Can you work these out from the model? Positions are in its coordinate system, mm. Face numbers are marked on the shaded views. Round coordinates to 2 decimals unless told otherwise and drop trailing zeros. Order: outer loops, then holes, each group sorted by start corner. A loop starts at its lowest first (then second) coordinate and runs counter-clockwise, first axis right, second up.
Q1. Will these pins go through, and if not, where does the flat tip stop? P1, Ø2, axis at x = -25, y = 5.5, coming from the +Z side (3 decimals); P2, Ø2, axis at x = 39, z = -13, coming from the -Y side; P3, Ø1, axis at x = 45, y = 1.5, coming from the -Z side (3 decimals); P4, Ø1, axis at x = -48, y = 2, coming from the +Z side (3 decimals).
Q2. If we section it at A-A (x = 22): Please give me the cut outline in (y, z) (3 decimals), plus the area to 3 significant figures.
Q3. If I drill on line 1 (X direction, y = 1.75, z = 24.5) (3 decimals); line 2 (Z direction, x = 4, y = 5.75) (3 decimals); line 3 (Z direction, x = -42.5, y = 4) (3 decimals), over which ranges is the centre line in solid material (lowest first)?
Q4. If we section it at B-B (y = 5.5): Please give me the cut outline in (x, z) (3 decimals), plus the area to 3 significant figures.
Q5. If we section it at D-D (x = 6): Please give me the cut outline in (y, z) (3 decimals), plus the area to 3 significant figures.
Q6. If we section it at C-C (z = -14): Please give me the cut outline in (x, y) (3 decimals), plus the area to 3 significant figures.
Q7. We'd pull the mould along Z, two halves only. Please class the marked faces 1 and 2: pulls with the +Z half, pulls with the -Z half, needs draft (parallel to the pull), parting line crosses it, or undercut.
from build123d import *

# Parameters (mm, degrees)
SKETCH1_W           = 7.75
SKETCH1_H           = 32.45
SKETCH1_H_2         = 7.9
SKETCH1_H_3         = 7.75
SKETCH1_W_2         = 16.15
SKETCH1_W_3         = 15.85
BOSS_EXTRUDE1_DEPTH = 3.2
SKETCH2_W           = 127.65
SKETCH2_H           = 6
BOSS_EXTRUDE2_DEPTH = 1
SKETCH3_W           = 127.65
SKETCH3_H           = 2.4
BOSS_EXTRUDE3_DEPTH = 5.4


with BuildPart() as part:
    # Sketch1 → Boss-Extrude1 (new body)
    with BuildSketch(Plane(origin=(0, 0, 0), x_dir=(1, 0, 0), z_dir=(0, 1, 0))):
        with Locations((-59.95, 0)):
            Rectangle(SKETCH1_W, SKETCH1_H)
        with Locations((-59.95, 20.175)):
            Rectangle(SKETCH1_W, SKETCH1_H_2)
        with Locations((-59.95, 28)):
            Rectangle(SKETCH1_W, SKETCH1_H_3)
        with Locations((-59.95, -20.175)):
            Rectangle(SKETCH1_W, SKETCH1_H_2)
        with Locations((-59.95, -28)):
            Rectangle(SKETCH1_W, SKETCH1_H_3)
        with Locations((-48, 20.175)):
            Rectangle(SKETCH1_W_2, SKETCH1_H_2)
        with Locations((-48, -20.175)):
            Rectangle(SKETCH1_W_2, SKETCH1_H_2)
        with Locations((-32, -28)):
            Rectangle(SKETCH1_W_3, SKETCH1_H_3)
        with Locations((-32, -20.175)):
            Rectangle(SKETCH1_W_3, SKETCH1_H_2)
        with Locations((-32, 0)):
            Rectangle(SKETCH1_W_3, SKETCH1_H)
        with Locations((-32, 20.175)):
            Rectangle(SKETCH1_W_3, SKETCH1_H_2)
        with Locations((-32, 28)):
            Rectangle(SKETCH1_W_3, SKETCH1_H_3)
        with Locations((-16, 20.175)):
            Rectangle(SKETCH1_W_2, SKETCH1_H_2)
        with Locations((-16, -20.175)):
            Rectangle(SKETCH1_W_2, SKETCH1_H_2)
        with Locations((0, -20.175)):
            Rectangle(SKETCH1_W_3, SKETCH1_H_2)
        with Locations((0, -28)):
            Rectangle(SKETCH1_W_3, SKETCH1_H_3)
        with Locations((0, 20.175)):
            Rectangle(SKETCH1_W_3, SKETCH1_H_2)
        Rectangle(SKETCH1_W_3, SKETCH1_H)
        with Locations((0, 28)):
            Rectangle(SKETCH1_W_3, SKETCH1_H_3)
        with Locations((32, 28)):
            Rectangle(SKETCH1_W_3, SKETCH1_H_3)
        with Locations((32, 20.175)):
            Rectangle(SKETCH1_W_3, SKETCH1_H_2)
        with Locations((32, 0)):
            Rectangle(SKETCH1_W_3, SKETCH1_H)
        with Locations((32, -20.175)):
            Rectangle(SKETCH1_W_3, SKETCH1_H_2)
        with Locations((32, -28)):
            Rectangle(SKETCH1_W_3, SKETCH1_H_3)
        with Locations((16, 20.175)):
            Rectangle(SKETCH1_W_2, SKETCH1_H_2)
        with Locations((16, -20.175)):
            Rectangle(SKETCH1_W_2, SKETCH1_H_2)
        with Locations((48, -20.175)):
            Rectangle(SKETCH1_W_2, SKETCH1_H_2)
        with Locations((48, 20.175)):
            Rectangle(SKETCH1_W_2, SKETCH1_H_2)
        with Locations((59.95, 28)):
            Rectangle(SKETCH1_W, SKETCH1_H_3)
        with Locations((59.95, 20.175)):
            Rectangle(SKETCH1_W, SKETCH1_H_2)
        with Locations((59.95, 0)):
            Rectangle(SKETCH1_W, SKETCH1_H)
        with Locations((59.95, -20.175)):
            Rectangle(SKETCH1_W, SKETCH1_H_2)
        with Locations((59.95, -28)):
            Rectangle(SKETCH1_W, SKETCH1_H_3)
    extrude(amount=BOSS_EXTRUDE1_DEPTH)

    # Sketch2 → Boss-Extrude2 (add)
    with BuildSketch(Plane(origin=(0, 3.2, 0), x_dir=(1, 0, 0), z_dir=(0, 1, 0))):
        with Locations((0, -20.175)):
            Rectangle(SKETCH2_W, SKETCH2_H)
        with Locations((0, 20.175)):
            Rectangle(SKETCH2_W, SKETCH2_H)
    extrude(amount=BOSS_EXTRUDE2_DEPTH)

    # Sketch3 → Boss-Extrude3 (add)
    with BuildSketch(Plane(origin=(0, 4.2, 0), x_dir=(1, 0, 0), z_dir=(0, 1, 0))):
        with Locations((0, 20.175)):
            Rectangle(SKETCH3_W, SKETCH3_H)
        with Locations((0, -20.175)):
            Rectangle(SKETCH3_W, SKETCH3_H)
    extrude(amount=BOSS_EXTRUDE3_DEPTH)


solid = part.part
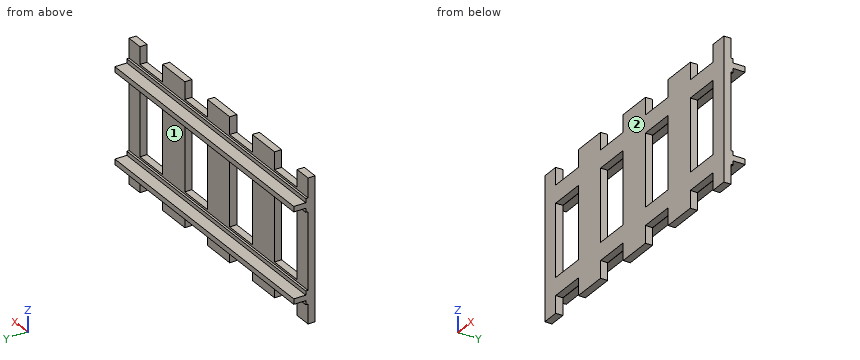
Solution:
1. P1: stops at z = 21.375
1. P2: stops at y = 0
1. P3: stops at z = -24.125
1. P4: stops at z = 24.125
2. outline: (0, -24.125) - (3.2, -24.125) - (3.2, -23.175) - (4.2, -23.175) - (4.2, -21.375) - (9.6, -21.375) - (9.6, -18.975) - (4.2, -18.975) - (4.2, -17.175) - (3.2, -17.175) - (3.2, -16.225) - (0, -16.225) - close; (0, 16.225) - (3.2, 16.225) - (3.2, 17.175) - (4.2, 17.175) - (4.2, 18.975) - (9.6, 18.975) - (9.6, 21.375) - (4.2, 21.375) - (4.2, 23.175) - (3.2, 23.175) - (3.2, 24.125) - (0, 24.125) - close
2. area: 88.5 mm2
3. line 1: x = -63.825 to -56.075, -39.925 to -24.075, -7.925 to 7.925, 24.075 to 39.925, 56.075 to 63.825
3. line 2: z = -21.375 to -18.975, 18.975 to 21.375
3. line 3: z = -23.175 to -17.175, 17.175 to 23.175
4. outline: (-63.825, -21.375) - (63.825, -21.375) - (63.825, -18.975) - (-63.825, -18.975) - close; (-63.825, 18.975) - (63.825, 18.975) - (63.825, 21.375) - (-63.825, 21.375) - close
4. area: 613 mm2
5. outline: (0, -31.875) - (3.2, -31.875) - (3.2, -23.175) - (4.2, -23.175) - (4.2, -21.375) - (9.6, -21.375) - (9.6, -18.975) - (4.2, -18.975) - (4.2, -17.175) - (3.2, -17.175) - (3.2, 17.175) - (4.2, 17.175) - (4.2, 18.975) - (9.6, 18.975) - (9.6, 21.375) - (4.2, 21.375) - (4.2, 23.175) - (3.2, 23.175) - (3.2, 31.875) - (0, 31.875) - close
5. area: 242 mm2
6. outline: (-63.825, 0) - (-56.075, 0) - (-56.075, 3.2) - (-63.825, 3.2) - close; (-39.925, 0) - (-24.075, 0) - (-24.075, 3.2) - (-39.925, 3.2) - close; (-7.925, 0) - (7.925, 0) - (7.925, 3.2) - (-7.925, 3.2) - close; (24.075, 0) - (39.925, 0) - (39.925, 3.2) - (24.075, 3.2) - close; (56.075, 0) - (63.825, 0) - (63.825, 3.2) - (56.075, 3.2) - close
6. area: 202 mm2
7. face 1: undercut
7. face 2: needs draft
